Part model, mm, in its own coordinate system. Face numbers are marked on the shaded views. A direction names the side the tool comes from. Coordinates: 2 decimals unless noted, no trailing zeros. Loops run counter-clockwise (first coordinate to the right, second up) from the corner with the lowest first, then second, coordinate; pieces in that order, holes last. Notation, with made-up numbers: M 2.25,2.5 L 43.25,2.5 A26 ccw 43.25,19.5 Z; hole C 46,29.25 d1. An arc over 180 degrees is marked long. Answer as a JSON object with one key per item and string values. Group by question number.
1. Drop flat-ended pins along their axis: pin 1 Ø4.5 at (x, z) = (-31.5, 2) entering from +Y; pin 2 Ø4 at (y, z) = (6, 0) entering from +X; pin 3 Ø1 at (y, z) = (1, -0.5) entering from +X. Give the stop position or say it passes through.
2. Drill centre lines: L1, parallel to X at y = 2.5, z = 8.75; L2, parallel to X at y = 4, z = 6.5; L3, parallel to Z at x = -36, y = 5.5. Where is each one in solid material? Low to high.
3. Saw through at A-A on z = 9. Write the cut outline in (x, y).
4. Mould opens along X. For the marked faces 1, 2 and 3 say: released by +X, released by -X, zero draft, split by the parting line, or undercut.
5. Saw through at B-B on x = -34.19. Write the cut outline in (y, z) (3 decimals).
6. 3-axis set-ups, long thin cutter, end or side, ignore diameter. For the marked faces 4, 5 and 6: which of +Z, -Z, +X, -X, +Y, -Y reach the whole face in a straight line?
7. Saw through at C-C on x = 26.5. Write the cut outline in (y, z).
from build123d import *

# Parameters (mm, degrees)
BOSS_EXTRUDE1_DEPTH             = 5
BOSS_EXTRUDE2_REACH             = 44.693
SKETCH2_W                       = 1
SKETCH2_H                       = 1.5
BOSS_EXTRUDE2_DIRECTION_2_REACH = 44.693
LPATTERN1_COUNT                 = 10
LPATTERN1_PITCH                 = 4.112759299
BOSS_EXTRUDE3_START             = 5
BOSS_EXTRUDE3_OUTLINE_R         = 5.875
BOSS_EXTRUDE3_DEPTH             = 2


# Read off the part's stored shape, not the designer's step: Boss-Extrude3
with BuildPart() as part:
    # Sketch1 → Boss-Extrude1 (new body)
    with BuildSketch(Plane(origin=(0, 0, 0), x_dir=(1, 0, 0), z_dir=(0, 1, 0))):
        with BuildLine():
            ThreePointArc((-38.901886937, -4.490905174), (-37.243453661, -13.019167833), (-28.907471708, -10.571093123))
            ThreePointArc((-28.907471708, -10.571093123), (-25.253097439, -6.507468715), (-20, -5))
            Line((-20, -5), (20, -5))
            ThreePointArc((20, -5), (25.253097439, -6.507468715), (28.907471708, -10.571093123))
            ThreePointArc((28.907471708, -10.571093123), (37.243453661, -13.019167833), (38.901886937, -4.490905174))
            ThreePointArc((38.901886937, -4.490905174), (30.575426833, 2.494044808), (20, 5))
            Line((20, 5), (-20, 5))
            ThreePointArc((-20, 5), (-30.575426833, 2.494044808), (-38.901886937, -4.490905174))
        make_face()
        Polygon((-31.913207445, -4.148110984), (-30.814488671, -6.096963409), (-29.715769982, -8.045815684), (-31.992562537, -11.8977047), (-36.466792555, -11.851889016), (-38.664230018, -7.954184316), (-36.387437463, -4.1022953), align=None, mode=Mode.SUBTRACT)
        Polygon((30.814488669, -6.096963413), (31.913207445, -4.148110984), (36.387437463, -4.1022953), (38.664230018, -7.954184316), (36.466792555, -11.851889016), (31.992562537, -11.8977047), (29.715769982, -8.045815684), align=None, mode=Mode.SUBTRACT)
    extrude(amount=BOSS_EXTRUDE1_DEPTH)

    # Boss-Extrude2: up to this face of the body (flat: up to its plane)
    boss_extrude2_end = Plane(part.part.faces().sort_by_distance((0, 2.5, 5))[0])
    # Sketch2 → Boss-Extrude2 (add, up to the picked face)
    with BuildSketch(Plane.XY, mode=Mode.PRIVATE) as boss_extrude2_sk1:
        with BuildLine():
            ThreePointArc((-19.507416847, 6.5), (-19.798015047, 5.582675362), (-20.563796496, 5))
            Line((-20.563796496, 5), (-18.507416847, 5))
            Line((-18.507416847, 5), (-18.507416847, 6.5))
            Line((-18.507416847, 6.5), (-19.507416847, 6.5))
        make_face()
    boss_extrude2_tool1 = split(extrude(boss_extrude2_sk1.sketch, amount=BOSS_EXTRUDE2_REACH, mode=Mode.PRIVATE), bisect_by=boss_extrude2_end, keep=Keep.BOTH, mode=Mode.PRIVATE)
    # Sketch2 → Boss-Extrude2 (add, up to the picked face)
    with BuildSketch(Plane.XY, mode=Mode.PRIVATE) as boss_extrude2_sk2:
        with Locations((-18.007416847, 5.75)):
            Rectangle(SKETCH2_W, SKETCH2_H)
    boss_extrude2_tool2 = split(extrude(boss_extrude2_sk2.sketch, amount=BOSS_EXTRUDE2_REACH, mode=Mode.PRIVATE), bisect_by=boss_extrude2_end, keep=Keep.BOTH, mode=Mode.PRIVATE)
    # Sketch2 → Boss-Extrude2 (add, up to the picked face)
    with BuildSketch(Plane.XY, mode=Mode.PRIVATE) as boss_extrude2_sk3:
        with BuildLine():
            Line((-17.507416847, 6.5), (-17.507416847, 5))
            Line((-17.507416847, 5), (-16.451037197, 5))
            ThreePointArc((-16.451037197, 5), (-17.216818646, 5.582675362), (-17.507416847, 6.5))
        make_face()
    boss_extrude2_tool3 = split(extrude(boss_extrude2_sk3.sketch, amount=BOSS_EXTRUDE2_REACH, mode=Mode.PRIVATE), bisect_by=boss_extrude2_end, keep=Keep.BOTH, mode=Mode.PRIVATE)
    # Sketch2 → Boss-Extrude2 (add, up to the picked face)
    with BuildSketch(Plane.XY, mode=Mode.PRIVATE) as boss_extrude2_sk4:
        with BuildLine():
            Line((-18.507416847, 8), (-18.507416847, 6.5))
            Line((-18.507416847, 6.5), (-17.507416847, 6.5))
            ThreePointArc((-17.507416847, 6.5), (-17.705365863, 7.338525492), (-18.257416847, 8))
            Line((-18.257416847, 8), (-18.507416847, 8))
        make_face()
    boss_extrude2_tool4 = split(extrude(boss_extrude2_sk4.sketch, amount=BOSS_EXTRUDE2_REACH, mode=Mode.PRIVATE), bisect_by=boss_extrude2_end, keep=Keep.BOTH, mode=Mode.PRIVATE)
    # Sketch2 → Boss-Extrude2 (add, up to the picked face)
    with BuildSketch(Plane.XY, mode=Mode.PRIVATE) as boss_extrude2_sk5:
        with BuildLine():
            ThreePointArc((-18.757416847, 8), (-19.30946783, 7.338525492), (-19.507416847, 6.5))
            Line((-19.507416847, 6.5), (-18.507416847, 6.5))
            Line((-18.507416847, 6.5), (-18.507416847, 8))
            Line((-18.507416847, 8), (-18.757416847, 8))
        make_face()
    boss_extrude2_tool5 = split(extrude(boss_extrude2_sk5.sketch, amount=BOSS_EXTRUDE2_REACH, mode=Mode.PRIVATE), bisect_by=boss_extrude2_end, keep=Keep.BOTH, mode=Mode.PRIVATE)
    boss_extrude2_1 = boss_extrude2_tool1.solids().sort_by(Axis((-19.182136, 5.660038, 0), (0, 0, 1)))[0]
    add(boss_extrude2_1)
    boss_extrude2_2 = boss_extrude2_tool2.solids().sort_by(Axis((-18.007417, 5.75, 0), (0, 0, 1)))[0]
    add(boss_extrude2_2)
    boss_extrude2_3 = boss_extrude2_tool3.solids().sort_by(Axis((-17.222958, 5.346083, 0), (0, 0, 1)))[0]
    add(boss_extrude2_3)
    boss_extrude2_4 = boss_extrude2_tool4.solids().sort_by(Axis((-18.090718, 7.135758, 0), (0, 0, 1)))[0]
    add(boss_extrude2_4)
    boss_extrude2_5 = boss_extrude2_tool5.solids().sort_by(Axis((-18.924116, 7.135758, 0), (0, 0, 1)))[0]
    add(boss_extrude2_5)
    boss_extrude2 = boss_extrude2_1 + boss_extrude2_2 + boss_extrude2_3 + boss_extrude2_4 + boss_extrude2_5  # Boss-Extrude2 as one shape, for the pattern or mirror that repeats it

    # Boss-Extrude2 direction 2: up to this face of the body (flat: up to its plane)
    boss_extrude2_direction_2_end = Plane(part.part.faces().sort_by_distance((0, 2.5, -5))[0])
    # Sketch2 → Boss-Extrude2 direction 2 (add, up to the picked face)
    with BuildSketch(Plane.XY, mode=Mode.PRIVATE) as boss_extrude2_direction_2_sk1:
        with BuildLine():
            ThreePointArc((-19.507416847, 6.5), (-19.798015047, 5.582675362), (-20.563796496, 5))
            Line((-20.563796496, 5), (-18.507416847, 5))
            Line((-18.507416847, 5), (-18.507416847, 6.5))
            Line((-18.507416847, 6.5), (-19.507416847, 6.5))
        make_face()
    boss_extrude2_direction_2_tool1 = split(extrude(boss_extrude2_direction_2_sk1.sketch, amount=-BOSS_EXTRUDE2_DIRECTION_2_REACH, mode=Mode.PRIVATE), bisect_by=boss_extrude2_direction_2_end, keep=Keep.BOTH, mode=Mode.PRIVATE)
    # Sketch2 → Boss-Extrude2 direction 2 (add, up to the picked face)
    with BuildSketch(Plane.XY, mode=Mode.PRIVATE) as boss_extrude2_direction_2_sk2:
        with Locations((-18.007416847, 5.75)):
            Rectangle(SKETCH2_W, SKETCH2_H)
    boss_extrude2_direction_2_tool2 = split(extrude(boss_extrude2_direction_2_sk2.sketch, amount=-BOSS_EXTRUDE2_DIRECTION_2_REACH, mode=Mode.PRIVATE), bisect_by=boss_extrude2_direction_2_end, keep=Keep.BOTH, mode=Mode.PRIVATE)
    # Sketch2 → Boss-Extrude2 direction 2 (add, up to the picked face)
    with BuildSketch(Plane.XY, mode=Mode.PRIVATE) as boss_extrude2_direction_2_sk3:
        with BuildLine():
            Line((-17.507416847, 6.5), (-17.507416847, 5))
            Line((-17.507416847, 5), (-16.451037197, 5))
            ThreePointArc((-16.451037197, 5), (-17.216818646, 5.582675362), (-17.507416847, 6.5))
        make_face()
    boss_extrude2_direction_2_tool3 = split(extrude(boss_extrude2_direction_2_sk3.sketch, amount=-BOSS_EXTRUDE2_DIRECTION_2_REACH, mode=Mode.PRIVATE), bisect_by=boss_extrude2_direction_2_end, keep=Keep.BOTH, mode=Mode.PRIVATE)
    # Sketch2 → Boss-Extrude2 direction 2 (add, up to the picked face)
    with BuildSketch(Plane.XY, mode=Mode.PRIVATE) as boss_extrude2_direction_2_sk4:
        with BuildLine():
            Line((-18.507416847, 8), (-18.507416847, 6.5))
            Line((-18.507416847, 6.5), (-17.507416847, 6.5))
            ThreePointArc((-17.507416847, 6.5), (-17.705365863, 7.338525492), (-18.257416847, 8))
            Line((-18.257416847, 8), (-18.507416847, 8))
        make_face()
    boss_extrude2_direction_2_tool4 = split(extrude(boss_extrude2_direction_2_sk4.sketch, amount=-BOSS_EXTRUDE2_DIRECTION_2_REACH, mode=Mode.PRIVATE), bisect_by=boss_extrude2_direction_2_end, keep=Keep.BOTH, mode=Mode.PRIVATE)
    # Sketch2 → Boss-Extrude2 direction 2 (add, up to the picked face)
    with BuildSketch(Plane.XY, mode=Mode.PRIVATE) as boss_extrude2_direction_2_sk5:
        with BuildLine():
            ThreePointArc((-18.757416847, 8), (-19.30946783, 7.338525492), (-19.507416847, 6.5))
            Line((-19.507416847, 6.5), (-18.507416847, 6.5))
            Line((-18.507416847, 6.5), (-18.507416847, 8))
            Line((-18.507416847, 8), (-18.757416847, 8))
        make_face()
    boss_extrude2_direction_2_tool5 = split(extrude(boss_extrude2_direction_2_sk5.sketch, amount=-BOSS_EXTRUDE2_DIRECTION_2_REACH, mode=Mode.PRIVATE), bisect_by=boss_extrude2_direction_2_end, keep=Keep.BOTH, mode=Mode.PRIVATE)
    boss_extrude2_direction_2_1 = boss_extrude2_direction_2_tool1.solids().sort_by(Axis((-19.182136, 5.660038, 0), (0, 0, -1)))[0]
    add(boss_extrude2_direction_2_1)
    boss_extrude2_direction_2_2 = boss_extrude2_direction_2_tool2.solids().sort_by(Axis((-18.007417, 5.75, 0), (0, 0, -1)))[0]
    add(boss_extrude2_direction_2_2)
    boss_extrude2_direction_2_3 = boss_extrude2_direction_2_tool3.solids().sort_by(Axis((-17.222958, 5.346083, 0), (0, 0, -1)))[0]
    add(boss_extrude2_direction_2_3)
    boss_extrude2_direction_2_4 = boss_extrude2_direction_2_tool4.solids().sort_by(Axis((-18.090718, 7.135758, 0), (0, 0, -1)))[0]
    add(boss_extrude2_direction_2_4)
    boss_extrude2_direction_2_5 = boss_extrude2_direction_2_tool5.solids().sort_by(Axis((-18.924116, 7.135758, 0), (0, 0, -1)))[0]
    add(boss_extrude2_direction_2_5)
    boss_extrude2_direction_2 = boss_extrude2_direction_2_1 + boss_extrude2_direction_2_2 + boss_extrude2_direction_2_3 + boss_extrude2_direction_2_4 + boss_extrude2_direction_2_5  # Boss-Extrude2 direction 2 as one shape, for the pattern or mirror that repeats it

    # LPattern1: Boss-Extrude2, Boss-Extrude2 direction 2 ×10
    with Locations(*[(i * LPATTERN1_PITCH, 0, 0) for i in range(1, LPATTERN1_COUNT)]):
        add(boss_extrude2)
        add(boss_extrude2_direction_2)

    # Boss-Extrude3 outline → Boss-Extrude3 (add)
    # profile 1 of 2: a face of its own
    with BuildSketch(Plane(origin=(0, 0, 0), x_dir=(1, 0, 0), z_dir=(0, 1, 0)).offset(BOSS_EXTRUDE3_START)):
        with Locations((34.19, -8)):
            Circle(BOSS_EXTRUDE3_OUTLINE_R)
        Polygon((36.466792555, -11.851889016), (31.992562537, -11.8977047), (29.715769982, -8.045815684), (31.913207445, -4.148110984), (36.387437463, -4.1022953), (38.664230018, -7.954184316), align=None, mode=Mode.SUBTRACT)
    # profile 2 of 2: a face of its own
    with BuildSketch(Plane(origin=(0, 0, 0), x_dir=(1, 0, 0), z_dir=(0, 1, 0)).offset(BOSS_EXTRUDE3_START)):
        with Locations((-34.19, -8)):
            Circle(BOSS_EXTRUDE3_OUTLINE_R)
        Polygon((-38.664230018, -7.954184316), (-36.387437463, -4.1022953), (-31.913207445, -4.148110984), (-29.715769982, -8.045815684), (-31.992562537, -11.8977047), (-36.466792555, -11.851889016), align=None, mode=Mode.SUBTRACT)
    extrude(amount=BOSS_EXTRUDE3_DEPTH)


solid = part.part
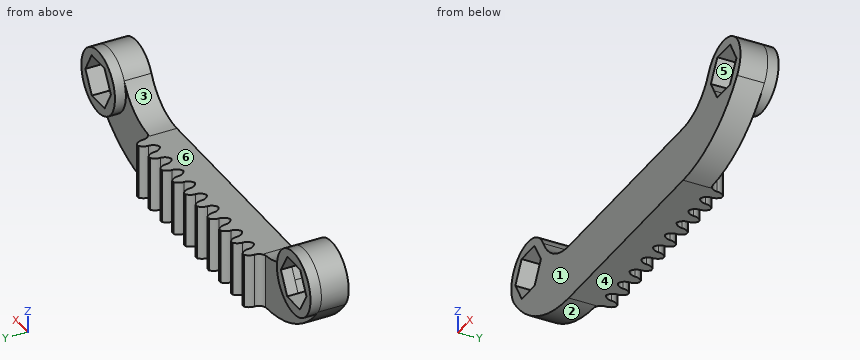
Outcome:
{
 "1": {"pin 1": "stops at y = 7", "pin 2": "stops at x = 36.49", "pin 3": "stops at x = 34.51"},
 "2": {"L1": "x = -40.02 to -38.22, -30.13 to -27.76, 27.76 to 30.13, 38.22 to 40.02", "L2": "x = -39.87 to -37.8, -30.59 to -25.24, 25.24 to 30.59, 37.8 to 39.87", "L3": "z = 2.41 to 4.11, 11.86 to 13.59"},
 "3": {"outline": "M -39.98,0 L -38.07,0 L -38.07,7 L -39.98,7 Z; M -30.28,0 L -27.95,0 L -27.95,5 L -28.4,5 L -28.4,7 L -30.28,7 Z; M 27.95,0 L 30.28,0 L 30.28,7 L 28.4,7 L 28.4,5 L 27.95,5 Z; M 38.07,0 L 39.98,0 L 39.98,7 L 38.07,7 Z"},
 "4": {"face 1": "zero draft", "face 2": "released by -X", "face 3": "undercut"},
 "5": {"outline": "M 0,-0.249 L 5,-0.249 L 5,2.125 L 7,2.125 L 7,4.125 L 0,4.125 Z; M 0,11.875 L 7,11.875 L 7,13.875 L 0,13.875 Z"},
 "6": {"face 4": "-Z, +X, -X, +Y, -Y", "face 5": "+Y, -Y", "face 6": "+Z, +Y, -Y"},
 "7": {"outline": "M 0,-4.09 L 5,-4.09 L 5,7.43 L 0,7.43 Z"}
}
